Geometry check sheet. Reference: drawing and pictorial views, mm from the part's lowest x, y, z. Give positions to 0.01 mm unless a question says otherwise; leave off trailing zeros. Order: outer loops, then holes, each group sorted by start corner. A loop starts at its lowest first (then second) coordinate and runs counter-clockwise, first axis right, second up.
Item 1: Gauge pin test, flat ends, axial feed: P1, Ø1.5, axis at y = 59.5, z = 2.5, coming from the -X side; P2, Ø1.8, axis at y = 130, z = 2.5, coming from the -X side; P3, Ø1.5, axis at x = 9, z = 3, coming from the -Y side (1 decimal); P4, Ø1.5, axis at x = 23.5, z = 2, coming from the +Y side. Record the tip position at first contact, or that the pin passes through.
Item 2: Material ranges on line 1 along Z through (x, y) = (16.8, 130); line 2 along X through (y, z) = (124.5, 0.3); line 3 along X through (y, z) = (117, 4.7), recorded low to high.
Item 3: Sectioned sample at A-A on y = 120.5. Record the boundary of the cut face in (x, z).
Item 4: Sectioned sample at C-C on y = 78.5. Record the boundary of the cut face in (x, z), and give its area (3 significant figures).
Item 5: Sectioned sample at B-B on z = 2.5. Count the separate pieces of the cut face and the enclosed holes in it, and give its area (3 significant figures).
Item 6: Release check for a two-part mould opening along Y. For the marked faces 1 and 2 record: released by +Y, released by -Y, zero draft, split by the parting line, or undercut.
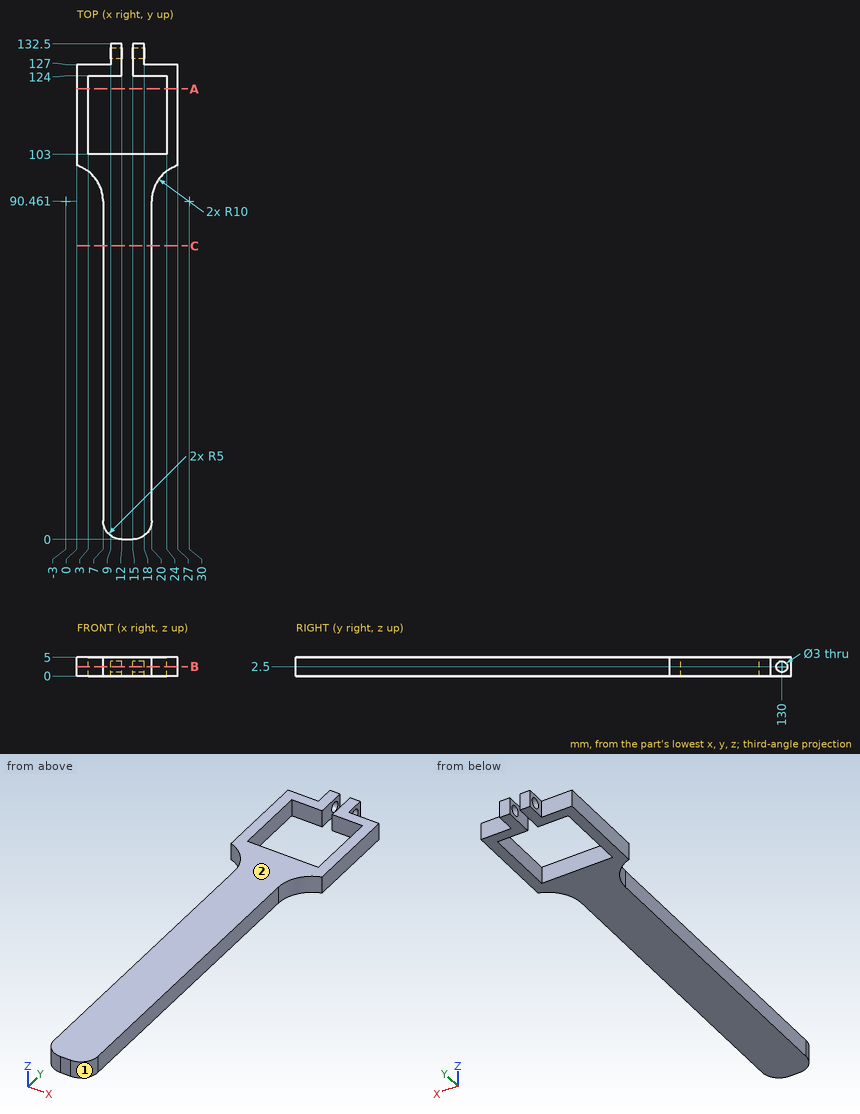
Report:
1. P1: stops at x = 7
1. P2: passes through
1. P3: stops at y = 0.5
1. P4: stops at y = 127
2. line 1: z = 0 to 1, 4 to 5
2. line 2: x = 0 to 12, 15 to 27
2. line 3: x = 0 to 3, 24 to 27
3. outline: (0, 0) - (3, 0) - (3, 5) - (0, 5) - close; (24, 0) - (27, 0) - (27, 5) - (24, 5) - close
4. outline: (7, 0) - (20, 0) - (20, 5) - (7, 5) - close
4. area: 65.0 mm2
5. separate pieces: 3
5. enclosed holes: 0
5. area: 1,620 mm2
6. face 1: released by -Y
6. face 2: zero draft
